Geometry: final body of the model. Coordinates: model frame, mm. Coordinates: 2 decimals unless noted, no trailing zeros. Order: outer loops, then holes, each group sorted by start corner. A loop starts at its lowest first (then second) coordinate and runs counter-clockwise, first axis right, second up. Notation, with made-up numbers: M 71,1.5 L 106,1.5 A13 ccw 106,7.5 Z; hole C -24.5,47 d2. An arc over 180 degrees is marked long. One line per question, with ' | ' between items.
from build123d import *

# Parameters (mm, degrees)
F0_R     = 0.75
F1_DEPTH = 1


# Not quite as in the source:
# - a feature names something its author has since deleted; it is built from what else it names


with BuildPart() as f1:
    # F0 (on Right) → F1 (new body)
    with BuildSketch(Plane.YZ):
        Polygon((8.384144865, 0), (0, 0), (0, -11.5), (11.5, -11.5), (11.5, 0), (10.38414, 0), (9.5, 0), align=None)
        with Locations((1.75, -9.75)):
            Circle(F0_R, mode=Mode.SUBTRACT)
        with Locations((1.75, -7.75)):
            Circle(F0_R, mode=Mode.SUBTRACT)
        with Locations((3.75, -9.75)):
            Circle(F0_R, mode=Mode.SUBTRACT)
        with Locations((3.75, -7.75)):
            Circle(F0_R, mode=Mode.SUBTRACT)
        with Locations((1.75, -5.75)):
            Circle(F0_R, mode=Mode.SUBTRACT)
        with Locations((1.75, -3.75)):
            Circle(F0_R, mode=Mode.SUBTRACT)
        with Locations((1.75, -1.75)):
            Circle(F0_R, mode=Mode.SUBTRACT)
        with Locations((3.75, -5.75)):
            Circle(F0_R, mode=Mode.SUBTRACT)
        with Locations((3.75, -3.75)):
            Circle(F0_R, mode=Mode.SUBTRACT)
        with Locations((3.75, -1.75)):
            Circle(F0_R, mode=Mode.SUBTRACT)
        with Locations((5.75, -9.75)):
            Circle(F0_R, mode=Mode.SUBTRACT)
        with Locations((7.75, -9.75)):
            Circle(F0_R, mode=Mode.SUBTRACT)
        with Locations((5.75, -7.75)):
            Circle(F0_R, mode=Mode.SUBTRACT)
        with Locations((7.75, -7.75)):
            Circle(F0_R, mode=Mode.SUBTRACT)
        with Locations((9.75, -9.75)):
            Circle(F0_R, mode=Mode.SUBTRACT)
        with Locations((9.75, -7.75)):
            Circle(F0_R, mode=Mode.SUBTRACT)
        with Locations((5.75, -5.75)):
            Circle(F0_R, mode=Mode.SUBTRACT)
        with Locations((5.75, -3.75)):
            Circle(F0_R, mode=Mode.SUBTRACT)
        with Locations((7.75, -5.75)):
            Circle(F0_R, mode=Mode.SUBTRACT)
        with Locations((7.75, -3.75)):
            Circle(F0_R, mode=Mode.SUBTRACT)
        with Locations((5.75, -1.75)):
            Circle(F0_R, mode=Mode.SUBTRACT)
        with Locations((7.75, -1.75)):
            Circle(F0_R, mode=Mode.SUBTRACT)
        with Locations((9.75, -5.75)):
            Circle(F0_R, mode=Mode.SUBTRACT)
        with Locations((9.75, -3.75)):
            Circle(F0_R, mode=Mode.SUBTRACT)
        with Locations((9.75, -1.75)):
            Circle(F0_R, mode=Mode.SUBTRACT)
    extrude(amount=F1_DEPTH)


solid = f1.part
1. Pin query (flat end, axial travel): P1, Ø1.2, axis at y = 5.75, z = -5.75, coming from the +X side. Return the tip coordinate at first contact, or that it passes through.
Response values:
P1: passes through
2. Section C-C, the plane x = 0.6. Give the number of separate pieces and of enclosed holes in the cut face, and give its area (3 significant figures).
Response values:
separate pieces: 1 | enclosed holes: 25 | area: 88.1 mm^2
3. Material intervals for line 1 (Z direction, x = 0.3, y = 3.75); line 2 (Z direction, x = 0.8, y = 5.25); line 3 (Y direction, x = 0.8, z = -4.25), sorted ascending. Write a range as [from, to].
Response values:
line 1: z = [-11.5, -10.5], [-9, -8.5], [-7, -6.5], [-5, -4.5], [-3, -2.5], [-1, 0] | line 2: z = [-11.5, -10.31], [-9.19, -8.31], [-7.19, -6.31], [-5.19, -4.31], [-3.19, -2.31], [-1.19, 0] | line 3: y = [0, 1.19], [2.31, 3.19], [4.31, 5.19], [6.31, 7.19], [8.31, 9.19], [10.31, 11.5]
4. Section B-B, the plane z = -1.75. Output: boundary loops of the cut face in (x, y).
Response values:
outline: M 0,0 L 1,0 L 1,1 L 0,1 Z; M 0,2.5 L 1,2.5 L 1,3 L 0,3 Z; M 0,4.5 L 1,4.5 L 1,5 L 0,5 Z; M 0,6.5 L 1,6.5 L 1,7 L 0,7 Z; M 0,8.5 L 1,8.5 L 1,9 L 0,9 Z; M 0,10.5 L 1,10.5 L 1,11.5 L 0,11.5 Z
5. Draft query along Y for faces 1 (the face through (0.493, 5.587, -4.482)), 2 (the face through (0.5, 11.5, -5.8)), 3 (the face through (0.5, 9, -3.7)), 4 (the face through (0.5, 0, -5.7)). Return one class per face: pulls with the +Y half, pulls with the -Y half, needs draft (parallel to the pull), parting line crosses it, or undercut.
Response values:
face 1: undercut | face 2: pulls with the +Y half | face 3: undercut | face 4: pulls with the -Y half
6. Section A-A, the plane y = 3.75. Output: boundary loops of the cut face in (x, z).
Response values:
outline: M 0,-11.5 L 1,-11.5 L 1,-10.5 L 0,-10.5 Z; M 0,-9 L 1,-9 L 1,-8.5 L 0,-8.5 Z; M 0,-7 L 1,-7 L 1,-6.5 L 0,-6.5 Z; M 0,-5 L 1,-5 L 1,-4.5 L 0,-4.5 Z; M 0,-3 L 1,-3 L 1,-2.5 L 0,-2.5 Z; M 0,-1 L 1,-1 L 1,0 L 0,0 Z
